```python
from build123d import *

# Parameters (mm, degrees)
BOSS_EXTRUDE1_DEPTH = 10
FILLET1_R           = 25


with BuildPart() as part:
    # Sketch1 → Boss-Extrude1 (new body)
    with BuildSketch(Plane.XY):
        Polygon((35, -75), (35, 50), (25, 50), (25, -50), (-25, -50), (-25, 50), (-35, 50), (-35, -75), align=None)
    extrude(amount=BOSS_EXTRUDE1_DEPTH)

    # Fillet1
    fillet1_edges = [part.edges().sort_by_distance(p)[0] for p in [
        (25, -50, 5),
        (-25, -50, 5),
    ]]
    fillet(fillet1_edges, radius=FILLET1_R - 0.0001)  # a hair under: the kernel refuses the full size


solid = part.part
```
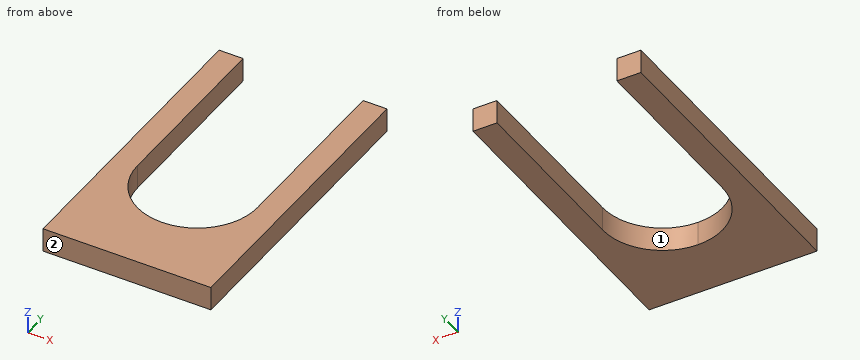
Geometry check sheet. Reference: the model listing, model coordinates, mm. Face numbers are marked on the shaded views. A direction names the side the tool comes from. Coordinates: 2 decimals unless noted, no trailing zeros. Order: outer loops, then holes, each group sorted by start corner. A loop starts at its lowest first (then second) coordinate and runs counter-clockwise, first axis right, second up.
Q1. Tool access check on the marked faces 1 and 2. Record the directions out of +Z, -Z, +X, -X, +Y, -Y that give a thin tool (end or side, any length) a straight path to the whole face; none if there is none.
Reply:
face 1: +Z, -Z, +Y
face 2: +Z, -Z, +X, -X, -Y
Q2. Sectioned sample at D-D on x = 23. Record the cut outline in (y, z), and give its area (3 significant figures).
Reply:
outline: (-75, 0) - (-34.8, 0) - (-34.8, 10) - (-75, 10) - close
area: 402 mm2
Q3. Sectioned sample at A-A on y = 21. Record the cut outline in (x, z), and give its area (3 significant figures).
Reply:
outline: (-35, 0) - (-25, 0) - (-25, 10) - (-35, 10) - close; (25, 0) - (35, 0) - (35, 10) - (25, 10) - close
area: 200 mm2
Q4. Sectioned sample at C-C on y = -46. Record the cut outline in (x, z), and give its area (3 significant figures).
Reply:
outline: (-35, 0) - (-13.56, 0) - (-13.56, 10) - (-35, 10) - close; (13.56, 0) - (35, 0) - (35, 10) - (13.56, 10) - close
area: 429 mm2
Q5. Thickness scan on probe 1 along X at (y, z) = (-17, 1.75); probe 2 along Y at (x, z) = (0, 6.5); probe 3 along X at (y, z) = (-48, 3.5). Record the ranges inside material, lowest first.
Reply:
probe 1: x = -35 to -25, 25 to 35
probe 2: y = -75 to -50
probe 3: x = -35 to -9.8, 9.8 to 35
Q6. Depth check by flat-ended pin: pin 1 Ø6 at (x, z) = (0, 1.5) entering from +Y. Enter the tip coordinate at first touch or a pass-through.
Reply:
pin 1: stops at y = -49.82
